```python
from build123d import *

# Parameters (mm, degrees)
SKETCH1_W           = 90
SKETCH1_H           = 50
SKETCH1_R           = 16
BOSS_EXTRUDE1_DEPTH = 6
SKETCH3_W           = 10
SKETCH3_H           = 50
BOSS_EXTRUDE2_DEPTH = 25
SCALE1_SCALE        = 7.5


with BuildPart() as part:
    # Sketch1 → Boss-Extrude1 (new body)
    with BuildSketch(Plane.XY):
        with Locations((45, 25)):
            Rectangle(SKETCH1_W, SKETCH1_H)
        with Locations((60, 22)):
            Circle(SKETCH1_R, mode=Mode.SUBTRACT)
    extrude(amount=BOSS_EXTRUDE1_DEPTH)

    # Sketch3 → Boss-Extrude2 (add)
    with BuildSketch(Plane(origin=(0, 0, 0), x_dir=(-1, 0, 0), z_dir=(0, 0, -1))):
        with Locations((-5, 25)):
            Rectangle(SKETCH3_W, SKETCH3_H)
    extrude(amount=BOSS_EXTRUDE2_DEPTH)


with BuildPart() as part_1:
    # Scale1: scaled about (28.492708796, 25.417495659, -2.587677502)
    add(part.part.scale(SCALE1_SCALE).moved(Location((-185.202607174, -165.213721784, 16.819903763))))


solid = part_1.part
```
CAD build for the part. Positions are in the model's coordinates, mm. A direction names the side the tool comes from. Round coordinates to 2 decimals unless told otherwise and drop trailing zeros. Write each loop counter-clockwise with the first axis right and the second up, starting at its lowest first coordinate (ties: lowest second). Pieces come first, ordered by that corner, then holes.
Item 1: Band-saw the part on D-D on z = -155. Write the cut outline in (x, y).
Filled in:
outline: (-185.2, -165.21) - (-110.2, -165.21) - (-110.2, 209.79) - (-185.2, 209.79) - close
Item 2: Band-saw the part on C-C on y = 186. Write the cut outline in (x, z).
Filled in:
outline: (-185.2, -170.68) - (-110.2, -170.68) - (-110.2, 16.82) - (489.8, 16.82) - (489.8, 61.82) - (-185.2, 61.82) - close
Item 3: Band-saw the part on A-A on y = 84. Write the cut outline in (x, z).
Filled in:
outline: (-185.2, -170.68) - (-110.2, -170.68) - (-110.2, 16.82) - (179.31, 16.82) - (179.31, 61.82) - (-185.2, 61.82) - close; (350.28, 16.82) - (489.8, 16.82) - (489.8, 61.82) - (350.28, 61.82) - close
Item 4: Drill centre lines: L1, parallel to Z at x = -46.5, y = -129.5; L2, parallel to X at y = 106.5, z = -105.5. Where is each one in solid material? Low to high.
Filled in:
L1: z = 16.82 to 61.82
L2: x = -185.2 to -110.2
Item 5: Tool access for faces 4 (the flat face through (-147, 25, -170.68)), 5 (the flat face through (119, 25, 16.82)): list every direction of +Z, -Z, +X, -X, +Y, -Y with a clear straight run to the whole face (end or side of a thin tool).
Filled in:
face 4: -Z, +X, -X, +Y, -Y
face 5: -Z, +X, +Y, -Y
Item 6: Mould opens along X. For faces 1 (the flat face through (148, 67, 61.82)), 2 (the cylindrical face through (144.913, 5.062, 39.005)), 3 (the flat face through (-110.203, 20, -76)) say: released by +X, released by -X, zero draft, split by the parting line, or undercut.
Filled in:
face 1: zero draft
face 2: undercut
face 3: released by +X
Item 7: Band-saw the part on B-B on x = 213. Write the cut outline in (y, z).
Filled in:
outline: (-165.21, 16.82) - (-108.46, 16.82) - (-108.46, 61.82) - (-165.21, 61.82) - close; (108.03, 16.82) - (209.79, 16.82) - (209.79, 61.82) - (108.03, 61.82) - close
Item 8: Drop flat-ended pins along their axis: pin 1 Ø1.5 at (y, z) = (-6.5, -55.5) entering from +X; pin 2 Ø1.5 at (x, y) = (369.5, 122) entering from -Z. Give the stop position or say it passes through.
Filled in:
pin 1: stops at x = -110.2
pin 2: stops at z = 16.82
